Geometry check sheet. Reference: the model listing, model coordinates, mm. Coordinates: 2 decimals unless noted, no trailing zeros. Loops run counter-clockwise (first coordinate to the right, second up) from the corner with the lowest first, then second, coordinate; pieces in that order, holes last.
from build123d import *

# Parameters (mm, degrees)
SKETCH_1_R      = 1.75
SKETCH_1_R_2    = 2
EXTRUDE_1_DEPTH = 3


with BuildPart() as part:
    # 草图1 → 凸台-拉伸1 (new body)
    with BuildSketch(Plane(origin=(0, 0, 0), x_dir=(1, 0, 0), z_dir=(0, 1, 0))):
        with BuildLine():
            Line((-20, 0), (-20, -69))
            Line((-20, -69), (20, -69))
            Line((20, -69), (20, 0))
            ThreePointArc((20, 0), (0, 20), (-20, 0))
        make_face()
        with Locations(Location((-6.5, 11.258330249, 0), (0, 0, 270))):
            Circle(SKETCH_1_R, mode=Mode.SUBTRACT)
        with Locations(Location((6.5, 11.258330249, 0), (0, 0, 270))):
            Circle(SKETCH_1_R, mode=Mode.SUBTRACT)
        with Locations(Location((-15.5, 0, 0), (0, 0, 270))):
            Circle(SKETCH_1_R, mode=Mode.SUBTRACT)
        with Locations(Location((15.5, 0, 0), (0, 0, 270))):
            Circle(SKETCH_1_R, mode=Mode.SUBTRACT)
        with Locations(Location((-6.5, -11.258330249, 0), (0, 0, 270))):
            Circle(SKETCH_1_R, mode=Mode.SUBTRACT)
        with Locations(Location((6.5, -11.258330249, 0), (0, 0, 270))):
            Circle(SKETCH_1_R, mode=Mode.SUBTRACT)
        with Locations(Location((-12.398128108, -34.265032361, 0), (0, 0, 270))):
            Circle(SKETCH_1_R_2, mode=Mode.SUBTRACT)
        with Locations(Location((-12.398128108, -60.734967639, 0), (0, 0, 270))):
            Circle(SKETCH_1_R_2, mode=Mode.SUBTRACT)
        with Locations(Location((12.398128108, -34.265032361, 0), (0, 0, 270))):
            Circle(SKETCH_1_R_2, mode=Mode.SUBTRACT)
        with Locations(Location((12.398128108, -60.734967639, 0), (0, 0, 270))):
            Circle(SKETCH_1_R_2, mode=Mode.SUBTRACT)
        with BuildLine():
            Line((3.394790848, 9.605209152), (3.394790848, -9.605209152))
            ThreePointArc((3.394790848, -9.605209152), (0, -13), (-3.394790848, -9.605209152))
            Line((-3.394790848, -9.605209152), (-3.394790848, 9.605209152))
            ThreePointArc((-3.394790848, 9.605209152), (0, 13), (3.394790848, 9.605209152))
        make_face(mode=Mode.SUBTRACT)
    extrude(amount=EXTRUDE_1_DEPTH)


solid = part.part
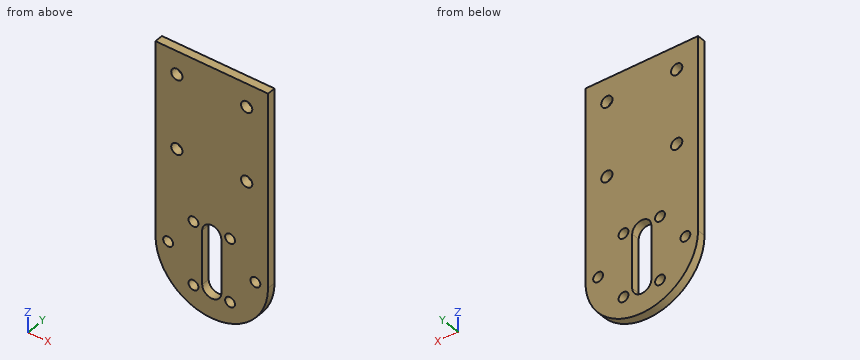
(1) Sectioned sample at C-C on x = -6.5. Record the cut outline in (y, z).
Findings:
outline: (0, -18.91) - (3, -18.91) - (3, -13.01) - (0, -13.01) - close; (0, -9.51) - (3, -9.51) - (3, 9.51) - (0, 9.51) - close; (0, 13.01) - (3, 13.01) - (3, 69) - (0, 69) - close
(2) Sectioned sample at A-A on x = 0. Record the cut outline in (y, z), and give its area (3 significant figures).
Findings:
outline: (0, -20) - (3, -20) - (3, -13) - (0, -13) - close; (0, 13) - (3, 13) - (3, 69) - (0, 69) - close
area: 189 mm2
(3) Scan lines: L1, parallel to X at y = 1.25, z = 0; L2, parallel to Z at x = 6, y = 1.9; L3, parallel to X at y = 0.95, z = 4.5. Record each from-to range of solid material in increasing order.
Findings:
L1: x = -20 to -17.25, -13.75 to -3.39, 3.39 to 13.75, 17.25 to 20
L2: z = -19.08 to -12.94, -9.58 to 9.58, 12.94 to 69
L3: x = -20 to -3.39, 3.39 to 20
(4) Sectioned sample at D-D on x = -15.5. Record the cut outline in (y, z), and give its area (3 significant figures).
Findings:
outline: (0, -12.64) - (3, -12.64) - (3, -1.75) - (0, -1.75) - close; (0, 1.75) - (3, 1.75) - (3, 69) - (0, 69) - close
area: 234 mm2
(5) Sectioned sample at B-B on y = 0.5. State how many separate pieces and enclosed holes the cut face has, and give its area (3 significant figures).
Findings:
separate pieces: 1
enclosed holes: 11
area: 3,110 mm2
(6) Gauge pin test, flat end, axial feed: pin 1 Ø1 at (x, y) = (4.5, 1) entering from -Z. Record the tip position at first contact, or that the pin passes through.
Findings:
pin 1: stops at z = -19.6
